Design review of the part built by this model. Coordinates are the model's own, in mm. A direction names the side the tool comes from. Coordinates: 2 decimals unless noted, no trailing zeros. Loops run counter-clockwise (first coordinate to the right, second up) from the corner with the lowest first, then second, coordinate; pieces in that order, holes last.
Q1. For P1, Ø9.5, axis at x = 78.53, y = -32.53, coming from the -Z side; P2, Ø1, axis at y = 79.5, z = 16.5, coming from the -X side; P3, Ø4, axis at x = -69.5, z = 5.5, coming from the +Y side; P4, Ø12, axis at x = -16.5, z = 6, coming from the -Y side, all flat-tipped, find the tip position at first contact; note any pin that passes through.
Q2. Draft analysis for pull direction X (two halves, no side actions). For faces 1 (the face through (95.38, -30.04, 10.87)), 2 (the face through (42, 1, 0)), 3 (the face through (-27.767, -74.879, 10.14)), 4 (the face through (27.767, 74.879, 10.14)), state which applies: released by +X, released by -X, zero draft, split by the parting line, or undercut.
Q3. Wall thickness on probe 1 along Y at (x, z) = (0, 4.85); probe 2 along Y at (x, z) = (80, 13); probe 3 along Y at (x, z) = (-28, 17.5): over which ranges is each line inside the solid? List them lowest first.
Q4. Add section A-A on y = 0. Give the boundary of the cut face in (x, z).
Q5. Add section C-C on z = 17.25. Give the number of separate pieces and of enclosed holes in the cut face, and give its area (3 significant figures).
Q6. Machinability: for faces 5 (the face through (26.984, -80.824, 10.14)), 6 (the face through (14.2, 31.2, 10)), which of the approach directions +Z, -Z, +X, -X, +Y, -Y give a long, thin tool a straight path to every point of the face, cutting with its end or side? Answer none if there is none.
Autodesk Inventor part; units mm, degrees
ref_plane "YZ Plane" through (0, 0, 0) normal (1, 0, 0) x (0, 1, 0)
ref_plane "XZ Plane" through (0, 0, 0) normal (0, 1, 0) x (-1, 0, 0)
ref_plane "XY Plane" through (0, 0, 0) normal (0, 0, 1) x (1, 0, 0)
sketch "Эскиз1" plane through (0, 0, 0) normal (0, 0, 1) x (1, 0, 0)
  circle A0 centre (0, 0) radius 32
  circle A1 centre (0, 0) radius 100
  dimension "d0" = 64
  dimension "d1" = 200
extrude "Выдавливание1" add sketch "Эскиз1" along normal blind 10
sketch "Эскиз2" plane through (0, 0, 10) normal (0, 0, 1) x (1, 0, 0)
  circle A0 centre (0, 0) radius 100
  circle A1 centre (0, 0) radius 70
  dimension "d4" = 140
extrude "Выдавливание2" add sketch "Эскиз2" along normal blind 10
fillet "Сопряжение1" radius 2 1 edges at (-70, 0, 10)
chamfer "Фаска1" distance 2 angle 45 2 edges at (-32, 0, 10) (-32, 0, 0)
sketch "Эскиз3" plane through (0, 0, 0) normal (0, 0, -1) x (-1, 0, 0)
  circle A0 centre (0, 0) radius 100
  line L0 (0, 0) -> (78.5298, 32.5281)
  line L1 (140, 0) -> (-140, 0)
  dimension "d11" = 85
  dimension "d12" = 22.5
hole "Отверстие1" at (-78.5298, 32.5281, 0) direction (0, 0, 1) diameter 12 end through all
pattern_circular "Круговой массив1" count 8 over 360 about axis through (0, 0, 1) along (0, 0, 1) of "Отверстие1"
chamfer "Фаска2" distance 2 angle 45 1 edges at (-100, 0, 0)
properties part number "Крышка перегородки12_CPY" material "Чугун, серый"
Entries:
1. P1: passes through
1. P2: stops at x = -61.31
1. P3: stops at y = 73.78
1. P4: stops at y = -99.45
2. face 1: split by the parting line
2. face 2: zero draft
2. face 3: undercut
2. face 4: undercut
3. probe 1: y = -100 to -32, 32 to 100
3. probe 2: y = -60 to -38.35, -26.71 to 26.71, 38.35 to 60
3. probe 3: y = -96 to -82.47, -74.59 to -64.16, 64.16 to 74.59, 82.47 to 96
4. outline: (-100, 2) - (-98, 0) - (-34, 0) - (-32, 2) - (-32, 8) - (-34, 10) - (-68, 10) arc R2 cw to (-70, 12) - (-70, 20) - (-100, 20) - close; (32, 2) - (34, 0) - (98, 0) - (100, 2) - (100, 20) - (70, 20) - (70, 12) arc R2 cw to (68, 10) - (34, 10) - (32, 8) - close
5. separate pieces: 1
5. enclosed holes: 9
5. area: 15,100 mm2
6. face 5: +Z, -Z
6. face 6: +Z
